Autodesk Fusion 360 part; units mm, degrees
sketch "Sketch1" plane through (0, 0, 0) normal (0, 0, 1) x (1, 0, 0)
  line L0 (0, 0) -> (0, 25.035) construction
  line L1 (0, 25.035) -> (12.9904, 17.535) construction
  circle A0 centre (12.9904, 17.535) radius 2.75
  line L2 (12.9904, 17.535) -> (17.0367, 24.5434) construction
  line L3 (8.6603, 20.035) -> (13.6603, 28.6952)
  line L4 (13.6603, 28.6952) -> (17.9904, 26.1952)
  line L5 (12.9904, 17.535) -> (15.372, 16.16) construction
  line L6 (17.3205, 15.035) -> (22.3205, 23.6952)
  line L7 (22.3205, 23.6952) -> (17.9904, 26.1952)
  line L8 (8.6603, 20.035) -> (3.6603, 11.3747)
  line L9 (3.6603, 11.3747) -> (7.9904, 8.8747)
  line L10 (17.3205, 15.035) -> (12.3205, 6.3747)
  line L11 (12.3205, 6.3747) -> (7.9904, 8.8747)
  line L12 (12.3205, 6.3747) -> (10.8205, 3.7766)
  line L13 (10.8205, 3.7766) -> (0, 10.0239)
  line L14 (0, 25.035) -> (0, 55.0088) construction
  line L15 (22.3205, 23.6952) -> (23.8205, 26.2933)
  line L16 (23.8205, 26.2933) -> (0, 40.0219)
  line L17 (-23.8205, 26.2933) -> (0, 40.0219)
  line L18 (-22.3205, 23.6952) -> (-23.8205, 26.2933)
  line L19 (-22.3205, 23.6952) -> (-17.9904, 26.1952)
  line L20 (-13.6603, 28.6952) -> (-17.9904, 26.1952)
  line L21 (-8.6603, 20.035) -> (-13.6603, 28.6952)
  line L22 (-8.6603, 20.035) -> (-3.6603, 11.3747)
  line L23 (-3.6603, 11.3747) -> (-7.9904, 8.8747)
  line L24 (-12.3205, 6.3747) -> (-7.9904, 8.8747)
  line L25 (-17.3205, 15.035) -> (-12.3205, 6.3747)
  line L26 (-17.3205, 15.035) -> (-22.3205, 23.6952)
  circle A1 centre (-12.9904, 17.535) radius 2.75
  line L27 (-12.3205, 6.3747) -> (-10.8205, 3.7766)
  line L28 (-10.8205, 3.7766) -> (0, 10.0239)
  dimension "d1" = 60
  dimension "d2" = 5.5
  dimension "d3" = 5
  dimension "d4" = 10
  dimension "d5" = 15
  dimension "d7" = 3
  dimension "d8" = 3
extrude "Extrude1" add sketch "Sketch1" along normal blind 26
sketch "Sketch2" plane through (-6.48, -3.7413, 0) normal (-0.866, -0.5, 0) x (0.5, -0.866, 0)
  line L0 (-34.6809, 0) -> (-8.6809, 0)
  line L1 (-8.6809, 0) -> (-8.6809, 26)
  line L2 (-8.6809, 26) -> (-34.6809, 26)
  line L3 (-34.6809, 26) -> (-34.6809, 0)
  line L4 (-34.6809, 26) -> (-8.6809, 0) construction
  line L5 (-31.9309, 23.25) -> (-11.4309, 23.25)
  line L6 (-11.4309, 23.25) -> (-11.4309, 2.75)
  line L7 (-11.4309, 2.75) -> (-31.9309, 2.75)
  line L8 (-31.9309, 2.75) -> (-31.9309, 23.25)
  line L9 (-31.9309, 23.25) -> (-11.4309, 2.75) construction
  line L10 (-11.4309, 23.25) -> (-31.9309, 2.75) construction
  point P0 (-21.6809, 13)
  dimension "d11" = 20.5
  dimension "d12" = 20.5
sketch "Sketch3" plane through (6.48, -3.7413, 0) normal (0.866, -0.5, 0) x (0.5, 0.866, 0)
  line L0 (8.6809, 0) -> (34.6809, 0)
  line L1 (34.6809, 0) -> (34.6809, 26)
  line L2 (34.6809, 26) -> (8.6809, 26)
  line L3 (8.6809, 26) -> (8.6809, 0)
  line L4 (8.6809, 26) -> (34.6809, 0) construction
  line L5 (31.9309, 23.25) -> (11.4309, 23.25)
  line L6 (11.4309, 23.25) -> (11.4309, 2.75)
  line L7 (11.4309, 2.75) -> (31.9309, 2.75)
  line L8 (31.9309, 2.75) -> (31.9309, 23.25)
  line L9 (31.9309, 23.25) -> (11.4309, 2.75) construction
  line L10 (11.4309, 23.25) -> (31.9309, 2.75) construction
  point P0 (21.6809, 13)
  dimension "d13" = 20.5
  dimension "d14" = 20.5
extrude "Extrude2" cut sketch "Sketch2" against normal blind 10 contours L5 L6 L7 L8
extrude "Extrude3" cut sketch "Sketch3" against normal blind 10 contours L5 L6 L7 L8
fillet "Fillet1" radius 3 1 edges at (0, 10.0239, 13)
fillet "Fillet2" radius 6 1 edges at (0, 40.0219, 13)
equation "d2 = screw"
equation "d5 = dist"
equation "d11 = slot"
equation "d12 = slot"
equation "d13 = slot"
equation "d14 = slot"
equation "dist = 15 mm"
equation "slot = 20.5 mm"
equation "screw = 5.5 mm"
Can you work these out from the model? Positions are in its coordinate system, mm. A direction names the side the tool comes from. Round coordinates to 2 decimals unless told otherwise and drop trailing zeros. Write each loop counter-clockwise with the first axis right and the second up, starting at its lowest first coordinate (ties: lowest second). Pieces come first, ordered by that corner, then holes. Notation, with made-up numbers: (4.25, 1) -> (40.25, 1) arc R23 ccw to (40.25, 27) -> close; hole circle Ø6 at (2, -3). An arc over 180 degrees is marked (long way). One line per question, with ' | ' between items. Start each with the question number.
1) If we mould it in two halves opening along X, with no side actions, what happens to faces 4 (the cylindrical face through (0.02, 9.56, 13.18)), 5 (the flat face through (-7.93, 8.62, 13.14)), 6 (the cylindrical face through (0.044, 39.097, 13.182)), 7 (the flat face through (7.93, 8.62, 13.14))? For each: released by +X, released by -X, zero draft, split by the parting line, or undercut.
2) Suppose I cut it at D-D on y = 14. Write out the boundary of the cut face in (x, z), then the cut area to 3 significant figures.
3) I need wall thicknesses on line 1 (X direction, y = 24.5, z = 12.75); line 2 (Z direction, x = -11, y = 23); line 3 (Y direction, x = 8, z = 14). Which ranges of each line are inside material? Lowest first, please. Write a range as [from, to].
4) I'm going to push flat-ended pins straight in: P1, Ø5, axis at x = 15, y = 14, coming from the -Z side; P2, Ø1, axis at x = 14, z = 3.5, coming from the +Y side; P3, Ø6, axis at x = -8, z = 12, coming from the -Y side; P4, Ø3.5, axis at x = 12.99, y = 17.54, coming from the +Z side. Where does each tip first touch, or does it pass through?
5) On a 3-axis mill with a long thin cutter (end or side, diameter ignored), from which of +Z, -Z, +X, -X, +Y, -Y can I reach the whole of each face in a straight line? I mean faces 1 (the flat face through (8.59, 19.91, 13.14)), 2 (the flat face through (-18.176, 26.377, 12.856)), 3 (the flat face through (6.226, 6.43, 12.818)). Say none if no direction works.
6) Suppose I cut it at C-C on z = 16. Write out the boundary of the cut face in (x, y).
7) Suppose I cut it at A-A on y = 8. Write out the boundary of the cut face in (x, z), then the cut area to 3 significant figures.
8) Suppose I cut it at B-B on x = -7.5. Write out the boundary of the cut face in (y, z), then the cut area to 3 significant figures.
Return value:
1) face 4: undercut | face 5: released by -X | face 6: split by the parting line | face 7: released by +X
2) outline: (-16.72, 0) -> (16.72, 0) -> (16.72, 2.75) -> (5.18, 2.75) -> (5.18, 23.25) -> (16.72, 23.25) -> (16.72, 26) -> (-16.72, 26) -> (-16.72, 23.25) -> (-5.18, 23.25) -> (-5.18, 2.75) -> (-16.72, 2.75) -> close | area: 396 mm2
3) line 1: x = [-22.79, -21.43], [-11.24, 11.24], [21.43, 22.79] | line 2: z = [0, 2.75], [23.25, 26] | line 3: y = [5.41, 8.58], [18.89, 35.41]
4) P1: stops at z = 0 | P2: stops at y = 32.24 | P3: stops at y = 3.78 | P4: passes through
5) face 1: none | face 2: -Y | face 3: +Z, -Z, -Y
6) outline: (-23.82, 26.29) -> (-22.45, 23.91) -> (-13.79, 28.91) -> (-3.54, 11.16) -> (-12.2, 6.16) -> (-10.82, 3.78) -> (-1.5, 9.16) arc R3 cw to (1.5, 9.16) -> (10.82, 3.78) -> (12.2, 6.16) -> (3.54, 11.16) -> (13.79, 28.91) -> (22.45, 23.91) -> (23.82, 26.29) -> (3, 38.3) arc R6 ccw to (-3, 38.3) -> close
7) outline: (-13.26, 0) -> (-3.51, 0) -> (-3.51, 26) -> (-13.26, 26) -> (-13.26, 23.25) -> (-9.01, 23.25) -> (-9.01, 2.75) -> (-13.26, 2.75) -> close; (3.51, 0) -> (13.26, 0) -> (13.26, 2.75) -> (9.01, 2.75) -> (9.01, 23.25) -> (13.26, 23.25) -> (13.26, 26) -> (3.51, 26) -> close | area: 333 mm2
8) outline: (5.69, 0) -> (35.7, 0) -> (35.7, 26) -> (5.69, 26) -> close; hole (8.87, 2.75) -> (18.03, 2.75) -> (18.03, 23.25) -> (8.87, 23.25) -> close | area: 592 mm2
